Geometry check sheet. Reference: the model listing, model coordinates, mm. A direction names the side the tool comes from. Round coordinates to 2 decimals unless told otherwise and drop trailing zeros. Write each loop counter-clockwise with the first axis right and the second up, starting at its lowest first coordinate (ties: lowest second). Pieces come first, ordered by that corner, then holes.
Item 1: Cross-section at B-B (x = -7). Enter the section's corners in (y, z).
Item 2: Cross-section at D-D (z = 20.25). Enter the section's corners in (x, y), then the cut area to 3 significant figures.
Item 3: Depth check by flat-ended pin: P1, Ø3, axis at y = 7.5, z = 21, coming from the -X side; P2, Ø3, axis at x = 2, y = 6, coming from the +Z side; P3, Ø6, axis at y = -0.5, z = 26.5, coming from the -X side. Enter the tip coordinate at first touch or a pass-through.
Item 4: Cross-section at A-A (x = 0). Enter the section's corners in (y, z), then the cut area to 3 significant figures.
Item 5: Draft check along X on faces 5 (the face through (-6.638, 0.72, 27.608)), 6 (the face through (3.5, 1, 21)), 7 (the face through (6.798, -20.014, 19.463)), 8 (the face through (-0.202, -20.014, 26.463)). Enter one of: pulls with the +X half, pulls with the -X half, needs draft (parallel to the pull), parting line crosses it, or undercut.
Item 6: Access from +Z, -Z, +X, -X, +Y, -Y to the whole of each face (thin tool, end or side, straight path). Record for faces 1 (the face through (-5.6, 0.72, 17.52)), 2 (the face through (5.57, 0.72, 17.55)), 3 (the face through (-3.5, 0.72, 26.62)), 4 (the face through (0, 1, 17.5)).
Item 7: Scan lines: probe 1 along X at (y, z) = (-19.65, 21); probe 2 along Z at (x, y) = (0, -20.2); probe 3 along Y at (x, z) = (6.25, 13.75). Record each from-to range of solid material in increasing order.
Item 8: Cross-section at C-C (y = 3.5). Enter the section's corners in (x, z), then the cut area to 3 significant figures.
from build123d import *

# Parameters (mm, degrees)
SKETCH1_R             = 10
SKETCH1_R_2           = 1.55
BOSS_EXTRUDE1_DEPTH   = 2
BOSS_EXTRUDE2_DEPTH   = 40
BODY_MOVE_COPY1_ANGLE = 90


with BuildPart() as part:
    # Sketch1 → Boss-Extrude1 (new body)
    with BuildSketch(Plane.XY):
        Circle(SKETCH1_R)
        with Locations((-7, 0)):
            Circle(SKETCH1_R_2, mode=Mode.SUBTRACT)
        with Locations((0, 7)):
            Circle(SKETCH1_R_2, mode=Mode.SUBTRACT)
        with Locations((0, -7)):
            Circle(SKETCH1_R_2, mode=Mode.SUBTRACT)
        with Locations((7, 0)):
            Circle(SKETCH1_R_2, mode=Mode.SUBTRACT)
    extrude(amount=BOSS_EXTRUDE1_DEPTH)

    # Sketch2 → Boss-Extrude2 (add)
    with BuildSketch(Plane.XY.offset(2)):
        Polygon((-1.378679656, -3.5), (1.378679656, -3.5), (5.603334512, -7.724654855), (7.724654855, -5.603334512), (3.5, -1.378679656), (3.5, 1.378679656), (7.705979833, 5.584659489), (5.584659489, 7.705979833), (1.378679656, 3.5), (-1.378679656, 3.5), (-5.520339389, 7.641659733), (-7.641659733, 5.520339389), (-3.5, 1.378679656), (-3.5, -1.378679656), (-7.683338011, -5.562017667), (-5.562017667, -7.683338011), align=None)
    extrude(amount=BOSS_EXTRUDE2_DEPTH)


with BuildPart() as part_1:
    # Body-Move/Copy1: moved
    add(part.part.rotate(Axis((0, 0, 21), (-1, 0, 0)), BODY_MOVE_COPY1_ANGLE))


solid = part_1.part
Resolved:
1. outline: (-21, 13.86) - (-19, 13.86) - (-19, 14.84) - (21, 14.84) - (21, 16.12) - (-19, 16.12) - (-19, 19.45) - (-21, 19.45) - close; (-21, 22.55) - (-19, 22.55) - (-19, 25.88) - (21, 25.88) - (21, 27.25) - (-19, 27.25) - (-19, 28.14) - (-21, 28.14) - close
2. outline: (-9.97, -21) - (-8.36, -21) - (-8.36, -19) - (-9.97, -19) - close; (-5.64, -21) - (5.64, -21) - (5.64, -19) - (3.5, -19) - (3.5, 21) - (-3.5, 21) - (-3.5, -19) - (-5.64, -19) - close; (8.36, -21) - (9.97, -21) - (9.97, -19) - (8.36, -19) - close
2. area: 309 mm2
3. P1: stops at x = -3.62
3. P2: stops at z = 26.62
3. P3: stops at x = -7.68
4. outline: (-21, 11) - (-19, 11) - (-19, 12.45) - (-21, 12.45) - close; (-21, 15.55) - (-19, 15.55) - (-19, 17.5) - (21, 17.5) - (21, 24.5) - (-19, 24.5) - (-19, 26.45) - (-21, 26.45) - close; (-21, 29.55) - (-19, 29.55) - (-19, 31) - (-21, 31) - close
4. area: 308 mm2
5. face 5: pulls with the -X half
5. face 6: pulls with the +X half
5. face 7: undercut
5. face 8: undercut
6. face 1: -X, +Y
6. face 2: +X, +Y
6. face 3: +Z, +Y
6. face 4: -Z, +Y
7. probe 1: x = -10 to -8.55, -5.45 to 5.45, 8.55 to 10
7. probe 2: z = 11 to 12.45, 15.55 to 26.45, 29.55 to 31
7. probe 3: y = -21 to -19
8. outline: (-7.68, 26.56) - (-3.5, 22.38) - (-3.5, 19.62) - (-7.64, 15.48) - (-5.52, 13.36) - (-1.38, 17.5) - (1.38, 17.5) - (5.58, 13.29) - (7.71, 15.42) - (3.5, 19.62) - (3.5, 22.38) - (7.72, 26.6) - (5.6, 28.72) - (1.38, 24.5) - (-1.38, 24.5) - (-5.56, 28.68) - close
8. area: 111 mm2
